```python
from build123d import *

# Parameters (mm, degrees)
SKETCH_1_W          = 25
SKETCH_1_H          = 32
EXTRUDE_1_DEPTH     = 2
SKETCH_2_W          = 21.5
SKETCH_2_H          = 27
EXTRUDE_2_DEPTH     = 18
SKETCH_3_W          = 1.5
SKETCH_3_H          = 28.5
EXTRUDE_3_DEPTH     = 29
SKETCH_4_W          = 21.5
SKETCH_4_H          = 1.5
EXTRUDE_4_DEPTH     = 11
SKETCH_6_R          = 2
EXTRUDE_5_DEPTH     = 11
SKETCH_7_W          = 6
SKETCH_7_H          = 1
EXTRUDE_6_DEPTH     = 11
SKETCH_8_R          = 1
CUT_EXTRUDE_1_DEPTH = 15
SKETCH_9_R          = 1
CUT_EXTRUDE_2_DEPTH = 5
CHAMFER_1_SIZE      = 1.5
SKETCH_10_W         = 20
SKETCH_10_H         = 25
CUT_EXTRUDE_3_DEPTH = 5
EXTRUDE_7_DEPTH     = 20


with BuildPart() as part:
    # Эскиз1 → Бобышка-Вытянуть1 (new body)
    with BuildSketch(Plane.XY):
        with Locations((12.5, 16)):
            Rectangle(SKETCH_1_W, SKETCH_1_H)
    extrude(amount=EXTRUDE_1_DEPTH)

    # Эскиз2 → Бобышка-Вытянуть2 (add)
    with BuildSketch(Plane.XY.offset(2)):
        with Locations((12.5, 16)):
            Rectangle(SKETCH_2_W, SKETCH_2_H)
    extrude(amount=EXTRUDE_2_DEPTH)

    # Эскиз3 → Бобышка-Вытянуть3 (add)
    with BuildSketch(Plane.XY.offset(2)):
        with Locations((12.5, 16)):
            Rectangle(SKETCH_3_W, SKETCH_3_H)
    extrude(amount=EXTRUDE_3_DEPTH)

    # Эскиз4 → Бобышка-Вытянуть4 (add)
    with BuildSketch(Plane.XY.offset(20)):
        with Locations((12.5, 20.75)):
            Rectangle(SKETCH_4_W, SKETCH_4_H)
    extrude(amount=EXTRUDE_4_DEPTH)

    # Эскиз6 → Бобышка-Вытянуть5 (add)
    with BuildSketch(Plane.XY.offset(31)):
        with Locations((12.5, 20.75)):
            Circle(SKETCH_6_R)
    extrude(amount=-EXTRUDE_5_DEPTH)

    # Эскиз7 → Бобышка-Вытянуть6 (add)
    with BuildSketch(Plane.XY.offset(20)):
        with Locations((7.002560395, 27)):
            Rectangle(SKETCH_7_W, SKETCH_7_H)
        with Locations((6.75, 4.25)):
            Rectangle(SKETCH_7_W, SKETCH_7_H)
        with Locations((7.002560395, 14.5)):
            Rectangle(SKETCH_7_W, SKETCH_7_H)
        with Locations((18.25, 4.25)):
            Rectangle(SKETCH_7_W, SKETCH_7_H)
        with Locations((17.997439605, 14.5)):
            Rectangle(SKETCH_7_W, SKETCH_7_H)
        with Locations((17.997439605, 27)):
            Rectangle(SKETCH_7_W, SKETCH_7_H)
    extrude(amount=EXTRUDE_6_DEPTH)

    # Эскиз8 → Вырез-Вытянуть1 (cut)
    with BuildSketch(Plane.XZ.offset(-3.75)):
        with Locations(Location((6.75, 27.5, 0), (0, 0, 270))):
            Circle(SKETCH_8_R)
        with Locations(Location((18.25, 27.5, 0), (0, 0, 270))):
            Circle(SKETCH_8_R)
    extrude(amount=-CUT_EXTRUDE_1_DEPTH, mode=Mode.SUBTRACT)

    # Эскиз9 → Вырез-Вытянуть2 (cut)
    with BuildSketch(Plane(origin=(0, 27.5, 0), x_dir=(1, 0, 0), z_dir=(0, 1, 0))):
        with Locations(Location((17.997439605, -27.5, 0), (0, 0, 270))):
            Circle(SKETCH_9_R)
        with Locations(Location((7.002560395, -27.5, 0), (0, 0, 270))):
            Circle(SKETCH_9_R)
    extrude(amount=-CUT_EXTRUDE_2_DEPTH, mode=Mode.SUBTRACT)

    # Фаска1
    chamfer_1_edges = [part.edges().sort_by_distance(p)[0] for p in [
        (4.002560395, 27, 31),
        (10.002560395, 27, 31),
        (9.75, 4.25, 31),
        (3.75, 4.25, 31),
        (10.002560395, 14.5, 31),
        (4.002560395, 14.5, 31),
        (21.25, 4.25, 31),
        (15.25, 4.25, 31),
        (20.997439605, 14.5, 31),
        (14.997439605, 14.5, 31),
        (14.997439605, 27, 31),
        (20.997439605, 27, 31),
    ]]
    chamfer(chamfer_1_edges, length=CHAMFER_1_SIZE)

    # Эскиз10 → Вырез-Вытянуть3 (cut)
    with BuildSketch(Plane(origin=(0, 0, 0), x_dir=(-1, 0, 0), z_dir=(0, 0, -1))):
        with Locations((-12.5, 16)):
            Rectangle(SKETCH_10_W, SKETCH_10_H)
    extrude(amount=-CUT_EXTRUDE_3_DEPTH, mode=Mode.SUBTRACT)

    # Эскиз12 → Бобышка-Вытянуть7 (add)
    with BuildSketch(Plane.ZY.offset(-22.5)):
        with BuildLine():
            Line((5, 5.26592597), (5, 26.73407403))
            ThreePointArc((5, 26.73407403), (-0.317848235, 28.452595927), (-5.853095184, 27.68196724))
            ThreePointArc((-5.853095184, 27.68196724), (-6.456920042, 27.028650367), (-6.301261639, 26.152752053))
            ThreePointArc((-6.301261639, 26.152752053), (-1.405439464, 16), (-0.568969813, 4.759547716))
            ThreePointArc((-0.568969813, 4.759547716), (-0.265824787, 3.923168323), (0.583761316, 3.659291744))
            ThreePointArc((0.583761316, 3.659291744), (2.86806198, 4.253205313), (5, 5.26592597))
        make_face()
    extrude(amount=EXTRUDE_7_DEPTH)


solid = part.part
```
Geometry: final body of the model. Coordinates: model frame, mm. A direction names the side the tool comes from. Round coordinates to 2 decimals unless told otherwise and drop trailing zeros. Loops run counter-clockwise (first coordinate to the right, second up) from the corner with the lowest first, then second, coordinate; pieces in that order, holes last. Notation, with made-up numbers: (63.25, -28.5) -> (68.25, -28.5) arc R13 cw to (68.25, -3.5) -> close; hole circle Ø1 at (63, -28.75). An arc over 180 degrees is marked (long way). Use one line per item in the form item = value. Start each with the question number.
1) Section C-C on y = 8.5. Output: boundary loops of the cut face in (x, z), then the cut area to 3 significant figures.
2) Section D-D on z = 27.5. Give the number of separate pieces and of enclosed holes in the cut face, then the cut area to 3 significant figures.
3) Access query for faces 1 (the flat face through (18, 15, 25)), 2 (the flat face through (14.997, 27, 25)), 3 (the cylindrical face through (7.426, 4.243, 28.237)), 4 (the flat face through (22.5, 28, 4)), 5 (the flat face through (12, 30.25, 16)). Directions: +Z, -Z, +X, -X, +Y, -Y. A direction counts if a zero-diameter tool reaches every point of the face in a straight line with its end or side. Return the directions, or none.
4) Section A-A on z = 16. Output: boundary loops of the cut face in (x, y), then the cut area to 3 significant figures.
5) Line query: L1, parallel to Y at x = 19.75, z = 26; L2, parallel to X at y = 14.2, z = 27.5; L3, parallel to Y at x = 8.5, z = 4. Output: solid intervals per line, ascending.
6) First-contact query: P1, Ø1.8, axis at x = 16.5, z = 24.5, coming from the +Y side; P2, Ø8.5, axis at y = 7, z = 18.5, coming from the -X side; P3, Ø5, axis at x = 16.5, z = 26.5, coming from the -Y side. Flat tips, straight axial feed; report the tip coordinate or a pass-through.
7) Draft query along X for faces 6 (the flat face through (2.5, 28, 4)), 7 (the flat face through (20.997, 27, 25)), 8 (the flat face through (19, 21.5, 25)), 9 (the flat face through (13.25, 10, 26)). Return one class per face: released by +X, released by -X, zero draft, split by the parting line, or undercut.
Response:
q1.outline = (0, 0) -> (2.5, 0) -> (2.5, -0.38) -> (22.5, -0.38) -> (22.5, 0) -> (25, 0) -> (25, 2) -> (23.25, 2) -> (23.25, 20) -> (13.25, 20) -> (13.25, 31) -> (11.75, 31) -> (11.75, 20) -> (1.75, 20) -> (1.75, 2) -> (0, 2) -> close
q1.area = 461 mm^2
q2.separate_pieces = 13
q2.enclosed_holes = 0
q2.area = 99.9 mm^2
q3.face_1 = +Z, +X
q3.face_2 = +Z, +Y
q3.face_3 = -Y
q3.face_4 = none
q3.face_5 = +Z, +X, -X, +Y
q4.outline = (1.75, 2.5) -> (11.75, 2.5) -> (11.75, 1.75) -> (13.25, 1.75) -> (13.25, 2.5) -> (23.25, 2.5) -> (23.25, 29.5) -> (13.25, 29.5) -> (13.25, 30.25) -> (11.75, 30.25) -> (11.75, 29.5) -> (1.75, 29.5) -> close
q4.area = 583 mm^2
q5.L1 = 3.75 to 4.75, 14 to 15, 20 to 21.5, 26.5 to 27.5
q5.L2 = 4 to 5.75, 7.75 to 10, 11.75 to 13.25, 15 to 17.25, 19.25 to 21
q5.L3 = 2.5 to 3.5, 4.73 to 27.27, 28.5 to 29.5
q6.P1 = 27.5
q6.P2 = 1.75
q6.P3 = 3.75
q7.face_6 = undercut
q7.face_7 = released by +X
q7.face_8 = zero draft
q7.face_9 = undercut
